Check sheet for the modelled part. Datum: model origin and axes. Units: mm. Face numbers are marked on the shaded views. A direction names the side the tool comes from. Coordinates: 2 decimals unless noted, no trailing zeros. Loops run counter-clockwise (first coordinate to the right, second up) from the corner with the lowest first, then second, coordinate; pieces in that order, holes last. Notation, with made-up numbers: M -24,26.5 L 16,26.5 A31 cw 16,53.5 Z; hole C 14.25,77.5 d10. An arc over 180 degrees is marked long. Return JSON: item names as keys, results as strings.
from build123d import *

# Parameters (mm, degrees)
SKETCH1_R           = 1.1
BOSS_EXTRUDE1_DEPTH = 1
BOSS_EXTRUDE2_DEPTH = 7.5


with BuildPart() as part:
    # Sketch1 → Boss-Extrude1 (new body)
    with BuildSketch(Plane.XY):
        with BuildLine():
            Line((0, 1.75), (-25.7, 1.75))
            Line((-25.7, 1.75), (-25.7, -9.25))
            Line((-25.7, -9.25), (-18.75, -9.25))
            Line((-18.75, -9.25), (-18.75, -17))
            ThreePointArc((-18.75, -17), (-18.237436867, -18.237436867), (-17, -18.75))
            Line((-17, -18.75), (0, -18.75))
            ThreePointArc((0, -18.75), (1.237436867, -18.237436867), (1.75, -17))
            Line((1.75, -17), (1.75, 0))
            ThreePointArc((1.75, 0), (1.237436867, 1.237436867), (0, 1.75))
        make_face()
        Circle(SKETCH1_R, mode=Mode.SUBTRACT)
        with Locations((-17, -17)):
            Circle(SKETCH1_R, mode=Mode.SUBTRACT)
    extrude(amount=BOSS_EXTRUDE1_DEPTH)

    # Sketch2 → Boss-Extrude2 (add)
    with BuildSketch(Plane.XY.offset(1)):
        with BuildLine():
            Line((-25.7, -9.25), (-18.72252415, -9.25))
            ThreePointArc((-18.72252415, -9.25), (-0.991671291, -15.477642868), (-8.5, 1.75))
            Line((-8.5, 1.75), (-25.7, 1.75))
            Line((-25.7, 1.75), (-25.7, -9.25))
        make_face()
    extrude(amount=BOSS_EXTRUDE2_DEPTH)


solid = part.part
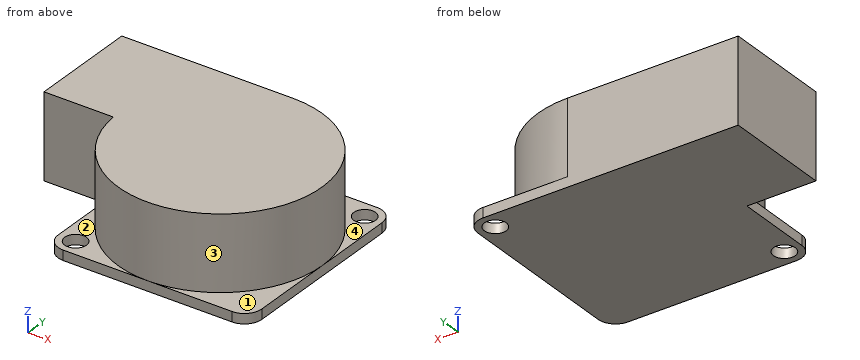
1) Go/stop test with flat-tipped pins: pin 1 Ø4 at (x, z) = (-22, 4) entering from -Y; pin 2 Ø1.1 at (y, z) = (-13.5, 0.5) entering from -X; pin 3 Ø3 at (x, y) = (0, 0) entering from +Z. Record where each tip stops, or that it passes through.
Answers:
{"pin 1": "y = -9.25", "pin 2": "x = -18.75", "pin 3": "z = 1"}
2) Set-up check for the marked faces 1, 2, 3 and 4: record each of +Z, -Z, +X, -X, +Y, -Y from which the full face is reachable in a straight line by a thin tool's end or side.
Answers:
{"face 1": "+Z, +X, -Y", "face 2": "+Z, -X, -Y", "face 3": "+Z", "face 4": "+Z, +X, +Y"}
3) Section check A-A on x = -16.25. Record the cut outline in (y, z), then the cut area to 3 significant figures.
Answers:
{"outline": "M -18.75,0 L -17.8,0 L -17.8,1 L -18.75,1 Z; M -16.2,0 L 1.75,0 L 1.75,8.5 L -15.21,8.5 L -15.21,1 L -16.2,1 Z", "area": "146 mm²"}
4) Section check C-C on z = 2. Record the cut outline in (x, y), then the cut area to 3 significant figures.
Answers:
{"outline": "M -25.7,-9.25 L -18.72,-9.25 A10.25 ccw long -8.5,1.75 L -25.7,1.75 Z", "area": "429 mm²"}
5) Section check B-B on y = -0.5. Record the cut outline in (x, z), then the cut area to 3 significant figures.
Answers:
{"outline": "M -25.7,0 L -0.98,0 L -0.98,1 L -2.09,1 L -2.09,8.5 L -25.7,8.5 Z; M 0.98,0 L 1.75,0 L 1.75,1 L 0.98,1 Z", "area": "203 mm²"}
6) Scan lines: line 1 along Y through (x, z) = (-17, 0.6); line 2 along Y through (x, z) = (-7.5, 7.5); line 3 along Y through (x, z) = (-16.25, 6). Record each from-to range of solid material in increasing order. Write a range as [from, to].
Answers:
{"line 1": "[-18.75, -18.1], [-15.9, 1.75]", "line 2": "[-18.7, 1.7]", "line 3": "[-15.21, 1.75]"}
7) Section check D-D on y = -12.5. Record the cut outline in (x, z).
Answers:
{"outline": "M -18.75,0 L 1.75,0 L 1.75,1 L 0.94,1 L 0.94,8.5 L -17.94,8.5 L -17.94,1 L -18.75,1 Z"}
